Read the model definition and answer for the solid it produces. Units are mm, in the model's axes. A direction names the side the tool comes from. Coordinates: 2 decimals unless noted, no trailing zeros. Write each loop counter-clockwise with the first axis right and the second up, starting at its lowest first coordinate (ties: lowest second). Pieces come first, ordered by that corner, then holes.
(1) Which of the six approach directions +Z, -Z, +X, -X, +Y, -Y give full straight-line access (tool end or side, diameter ignored) to faces 5 (the flat face through (2, 17.7, 5)), 6 (the flat face through (-7.624, -3, 5))?
(2) Section C-C on z = 86 is taken. Write down the section's boundary in (x, y), then the cut area to 3 significant figures.
(3) The mould has two halves that part along X. Classify faces 1 (the cylindrical face through (13.04, -4.82, 1.91)), 2 (the flat face through (14.601, -2, 5)), 3 (the flat face through (11.426, -3, 5)), 4 (the flat face through (2, -29.925, 5)): +X half, -X half, draft (parallel to the pull), parting line (faces both ways), or undercut.
(4) Find the intervals of material crossed by probe 1 along X at (y, z) = (-19.5, -288); probe 2 along Y at (x, z) = (6.5, -216); probe 3 along Z at (x, y) = (12.5, -8.5), in increasing order.
(5) Section A-A on z = 0 is taken. Write down the section's boundary in (x, y).
(6) Section B-B on x = 2.5 is taken. Write down the section's boundary in (y, z), then the cut area to 3 significant figures.
from build123d import *

# Parameters (mm, degrees)
SKETCH1_W           = 25.4
SKETCH1_H           = 50.8
SKETCH1_W_2         = 19.05
SKETCH1_H_2         = 44.45
BOSS_EXTRUDE1_DEPTH = 381
SKETCH2_R           = 6.35
CUT_EXTRUDE1_DEPTH  = 25.4


with BuildPart() as part:
    # Sketch1 → Boss-Extrude1 (new, symmetric)
    with BuildSketch(Plane.XY):
        with Locations((1.901454405, -7.699719174)):
            Rectangle(SKETCH1_W, SKETCH1_H)
        with Locations((1.901454405, -7.699719174)):
            Rectangle(SKETCH1_W_2, SKETCH1_H_2, mode=Mode.SUBTRACT)
    extrude(amount=BOSS_EXTRUDE1_DEPTH, both=True)

    # Sketch2 → Cut-Extrude1 (cut)
    with BuildSketch(Plane(origin=(14.601454405, 0, 0), x_dir=(0, 0, -1), z_dir=(1, 0, 0))):
        with Locations(Location((0, -10.874719174, 0), (0, 0, 90))):
            Circle(SKETCH2_R)
    extrude(amount=-CUT_EXTRUDE1_DEPTH, mode=Mode.SUBTRACT)


solid = part.part
Response:
1. face 5: +Z, -Z, +X, -X, +Y
1. face 6: +Z, -Z
2. outline: (-10.8, -33.1) - (14.6, -33.1) - (14.6, 17.7) - (-10.8, 17.7) - close; hole (-7.62, -29.92) - (11.43, -29.92) - (11.43, 14.53) - (-7.62, 14.53) - close
2. area: 444 mm2
3. face 1: draft
3. face 2: +X half
3. face 3: undercut
3. face 4: undercut
4. probe 1: x = -10.8 to -7.62, 11.43 to 14.6
4. probe 2: y = -33.1 to -29.92, 14.53 to 17.7
4. probe 3: z = -381 to -5.89, 5.89 to 381
5. outline: (-10.8, -33.1) - (14.6, -33.1) - (14.6, -17.22) - (11.43, -17.22) - (11.43, -29.92) - (-7.62, -29.92) - (-7.62, -17.22) - (-10.8, -17.22) - close; (-10.8, -4.52) - (-7.62, -4.52) - (-7.62, 14.53) - (11.43, 14.53) - (11.43, -4.52) - (14.6, -4.52) - (14.6, 17.7) - (-10.8, 17.7) - close
6. outline: (-33.1, -381) - (-29.92, -381) - (-29.92, 381) - (-33.1, 381) - close; (14.53, -381) - (17.7, -381) - (17.7, 381) - (14.53, 381) - close
6. area: 4,840 mm2
